from build123d import *

# Parameters (mm, degrees)
EXTRUDE_1_DEPTH     = 100
CUT_EXTRUDE_2_DEPTH = 103.22383051
FILLET_2_R          = 5
CHAMFER_1_SIZE      = 1


with BuildPart() as part:
    # 草图2 → 凸台-拉伸1 (new body)
    with BuildSketch(Plane.XY):
        with BuildLine():
            Line((1.5, 4.769696007), (1.5, 15))
            Line((1.5, 15), (4, 15))
            Line((4, 15), (4, 3))
            ThreePointArc((4, 3), (4.330127019, -2.5), (-0.598076211, -4.964101615))
            Line((-0.598076211, -4.964101615), (-10.990381057, -10.964101615))
            Line((-10.990381057, -10.964101615), (-12.240381057, -8.799038106))
            Line((-12.240381057, -8.799038106), (-3.38067791, -3.683886109))
            ThreePointArc((-3.38067791, -3.683886109), (-4.330127019, -2.5), (-4.88067791, -1.085809898))
            Line((-4.88067791, -1.085809898), (-13.740381057, -6.200961894))
            Line((-13.740381057, -6.200961894), (-14.990381057, -4.035898385))
            Line((-14.990381057, -4.035898385), (-4.598076211, 1.964101615))
            ThreePointArc((-4.598076211, 1.964101615), (-4.330127019, 2.5), (-4, 3))
            Line((-4, 3), (-4, 15))
            Line((-4, 15), (-1.5, 15))
            Line((-1.5, 15), (-1.5, 4.769696007))
            ThreePointArc((-1.5, 4.769696007), (0, 5), (1.5, 4.769696007))
        make_face()
    extrude(amount=EXTRUDE_1_DEPTH)

    # 草图5 → 切除-拉伸2 (cut, through all)
    with BuildSketch(Plane.XY.offset(100)):
        with BuildLine():
            Line((4, 3), (-0.598076211, -4.964101615))
            ThreePointArc((-0.598076211, -4.964101615), (4.330127019, -2.5), (4, 3))
        make_face()
    extrude(amount=-CUT_EXTRUDE_2_DEPTH, mode=Mode.SUBTRACT)

    # 圆角2
    fillet_2_edges = [part.edges().sort_by_distance(p)[0] for p in [
        (4, 3, 50),
        (-0.598076211, -4.964101615, 50),
        (-4.598076211, 1.964101615, 50),
    ]]
    fillet(fillet_2_edges, radius=FILLET_2_R)

    # 倒角1
    chamfer_1_edges = [part.edges().sort_by_distance(p)[0] for p in [
        (-1.5, 15, 50),
        (1.5, 15, 50),
        (-12.240381057, -8.799038106, 50),
        (-13.740381057, -6.200961894, 50),
    ]]
    chamfer(chamfer_1_edges, length=CHAMFER_1_SIZE)


solid = part.part
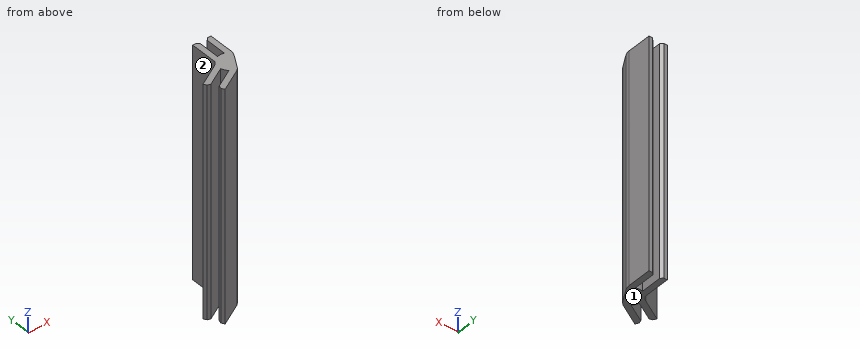
Source: CAD feature listing. Evaluate the final solid. Frame: model axes, mm. Face numbers are marked on the shaded views. A direction names the side the tool comes from. Give positions to 0.01 mm unless a question says otherwise; leave off trailing zeros. Loops run counter-clockwise (first coordinate to the right, second up) from the corner with the lowest first, then second, coordinate; pieces in that order, holes last. Notation, with made-up numbers: (58, -14.75) -> (95, -14.75) arc R22 cw to (95, 6.25) -> close; hole circle Ø1 at (14, -36.5). An arc over 180 degrees is marked (long way). Use a Markdown table: item, result. Add a question column.
1) Section query A-A, the plane y = 6.5. Return the cut outline in (x, z).
2) Reachability of the marked faces 1 and 2 from +Z, -Z, +X, -X, +Y, -Y: full face, straight path, thin tool, end or side. Return the list, or none.
3) Section query B-B, the plane z = 9.5. Return the cut outline in (x, y), then the cut area to 3 significant figures.
4) First-contact query: pin 1 (4 mm diameter, centred on x = -11.5, z = 42.5, fed in from +Y); pin 2 (1 mm diameter, centred on y = 2.5, z = 77, fed in from +X); pin 3 (10 mm diameter, centred on y = -1.5, z = 30.5, fed in from +X); pin 4 (8 mm diameter, centred on y = -1, z = 37.5, fed in from -X). Flat tips, straight axial feed; report the tip coordinate or a pass-through.
5) Section query C-C, the plane x = -8. Return the cut outline in (y, z).
6) Line query: line 1 along X through (y, z) = (12.75, 73); line 2 along Y through (x, z) = (-8.5, 15.5); line 3 along Y through (x, z) = (-10.25, 9). Output: solid intervals per line, ascending. Write a range as [from, to].
Numbers:
| question | item | result |
|---|---|---|
| 1 | outline | (-4, 0) -> (-1.5, 0) -> (-1.5, 100) -> (-4, 100) -> close; (1.5, 0) -> (4, 0) -> (4, 100) -> (1.5, 100) -> close |
| 2 | face 1 | -Z, +X, -X, +Y, -Y |
| 2 | face 2 | +Z, -Z, -X, +Y |
| 3 | outline | (-14.99, -4.04) -> (-14.24, -5.33) -> (-12.87, -5.7) -> (-4.88, -1.09) arc R5 ccw to (-3.38, -3.68) -> (-11.37, -8.3) -> (-11.74, -9.67) -> (-10.99, -10.96) -> (-1.76, -5.63) arc R5 ccw to (0.07, -3.8) -> (3.33, 1.84) arc R5 ccw to (4, 4.34) -> (4, 15) -> (2.5, 15) -> (1.5, 14) -> (1.5, 4.77) arc R5 ccw to (-1.5, 4.77) -> (-1.5, 14) -> (-2.5, 15) -> (-4, 15) -> (-4, 3) arc R5 ccw to (-4.14, 2.81) arc R5 cw to (-5.77, 1.28) -> close |
| 3 | area | 165 mm2 |
| 4 | pin 1 | stops at y = -0.87 |
| 4 | pin 2 | stops at x = 3.82 |
| 4 | pin 3 | stops at x = 3.93 |
| 4 | pin 4 | stops at x = -14.99 |
| 5 | outline | (-9.24, 0) -> (-6.35, 0) -> (-6.35, 100) -> (-9.24, 100) -> close; (-2.89, 0) -> (0, 0) -> (0, 100) -> (-2.89, 100) -> close |
| 6 | line 1 | x = [-4, -1.5], [1.5, 4] |
| 6 | line 2 | y = [-9.53, -6.64], [-3.18, -0.29] |
| 6 | line 3 | y = [-10.54, -7.65], [-4.19, -1.3] |
